Input: dimensioned drawing with shaded views. Units: mm. Origin: part minimum x, y, z. A direction names the side the tool comes from. Round coordinates to 2 decimals unless told otherwise and drop trailing zeros. Order: outer loops, then holes, each group sorted by start corner. A loop starts at its lowest first (then second) coordinate and runs counter-clockwise, first axis right, second up. Notation, with made-up numbers: (75, 27.25) - (125, 27.25) arc R13 cw to (125, 33.25) - close; hole circle Ø9 at (-33, 87.25). An arc over 180 degrees is marked (long way). Return JSON: item names as keys, results as strings. Group by question number.
1) Access query for the marked faces 1 and 2. Directions: +Z, -Z, +X, -X, +Y, -Y. A direction counts if a zero-diameter tool reaches every point of the face in a straight line with its end or side. Return the directions, or none.
2) Section C-C, the plane z = 21.5. Return loops of the section in (x, y).
3) Contact query for flat-ended pins moving along their axis: P1, Ø2, axis at x = 2, z = 26.5, coming from the +Y side; P2, Ø2, axis at x = 6.5, y = 5.5, coming from the -Z side. Output: stop coordinate, or through.
4) Section A-A, the plane y = 3. Return loops of the section in (x, z) (1 decimal).
5) Section D-D, the plane z = 32.5. Return loops of the section in (x, y).
6) Ray query, line 1 (Z direction, x = 4.75, y = 5); line 2 (Z direction, x = 2, y = 1.5); line 3 (X direction, y = 3.75, z = 32). Return the intervals inside material, ascending. Write a range as from..to.
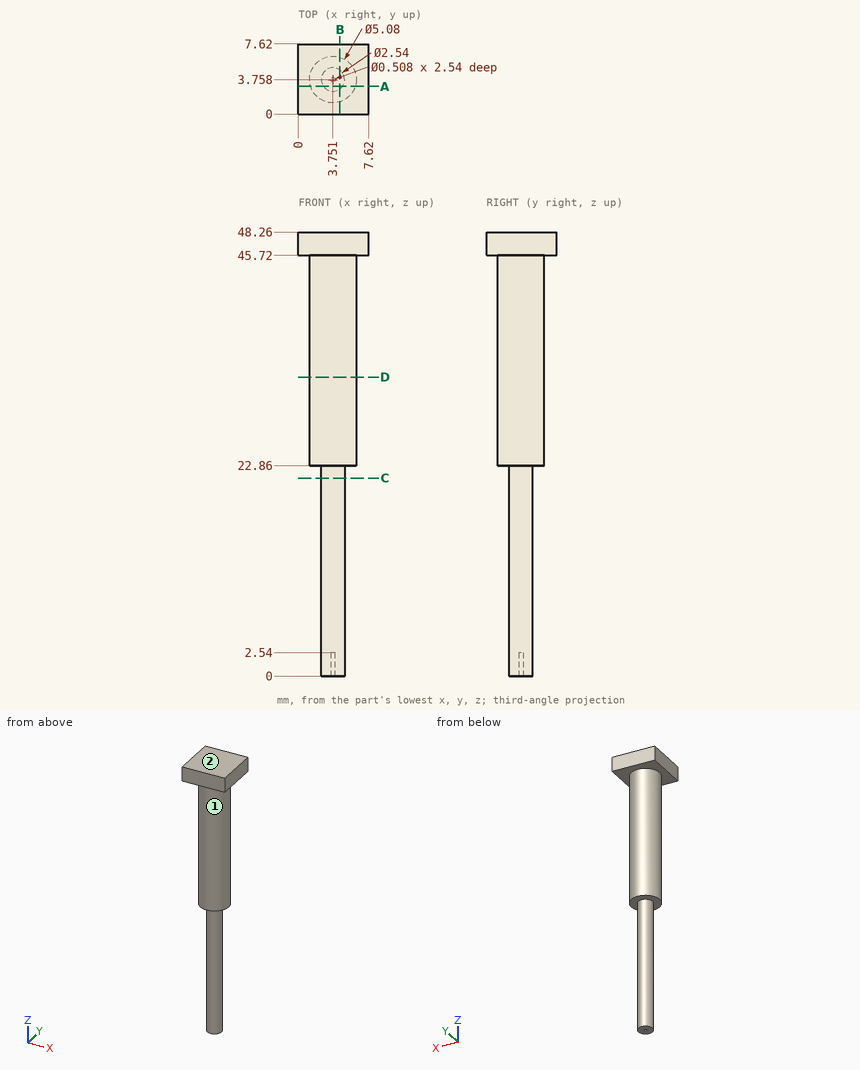
Geometry check:
{
 "1": {"face 1": "-Z", "face 2": "+Z, +X, -X, +Y, -Y"},
 "2": {"outline": "circle Ø2.54 at (3.75, 3.76)"},
 "3": {"P1": "y = 6.18", "P2": "z = 22.86"},
 "4": {"outline": "(0, 45.7) - (1.3, 45.7) - (1.3, 22.9) - (2.7, 22.9) - (2.7, 0) - (4.8, 0) - (4.8, 22.9) - (6.2, 22.9) - (6.2, 45.7) - (7.6, 45.7) - (7.6, 48.3) - (0, 48.3) - close"},
 "5": {"outline": "circle Ø5.08 at (3.75, 3.76)"},
 "6": {"line 1": "22.86..48.26", "line 2": "45.72..48.26", "line 3": "1.21..6.29"}
}
